Here's how the part is built. I have some questions about the finished solid (model axes, mm). A direction names the side the tool comes from. Give positions to 0.01 mm unless a question says otherwise; leave off trailing zeros. Order: outer loops, then holes, each group sorted by start corner. A loop starts at its lowest first (then second) coordinate and runs counter-clockwise, first axis right, second up. Notation, with made-up numbers: M 67,78.25 L 96,78.25 A17 ccw 96,95.25 Z; hole C -23,-10 d8. An arc over 180 degrees is marked long. One line per item, written item: value. Start each with the question number.
Autodesk Inventor part; units mm, degrees
ref_plane "YZ Plane" through (0, 0, 0) normal (1, 0, 0) x (0, 1, 0)
ref_plane "XZ Plane" through (0, 0, 0) normal (0, 1, 0) x (-1, 0, 0)
ref_plane "XY Plane" through (0, 0, 0) normal (0, 0, 1) x (1, 0, 0)
sketch "Sketch1" plane through (0, 0, 0) normal (0, 1, 0) x (-1, 0, 0)
  circle A0 centre (0, 0) radius 14
  dimension "d0" = 28
extrude "Extrusion1" add sketch "Sketch1" along normal blind 19
sketch "Sketch3" plane through (0, 19, 0) normal (0, 1, 0) x (1, 0, 0)
  circle A0 centre (0, 0) radius 14
  line L0 (3.5, 13.5554) -> (3.5, 17.5)
  arc A1 (3.5, 17.5) -> (-3.5, 17.5) centre (0, 17.5) ccw
  line L1 (-3.5, 17.5) -> (-3.5, 13.5554)
  arc A2 (3.5, 13.5554) -> (-3.5, 13.5554) centre (0, 0) ccw
  circle A3 centre (0, 17.5) radius 2
  line L2 (-3.5, -13.5554) -> (-3.5, -17.5)
  arc A4 (-3.5, -17.5) -> (3.5, -17.5) centre (0, -17.5) ccw
  line L3 (3.5, -17.5) -> (3.5, -13.5554)
  arc A5 (-3.5, -13.5554) -> (3.5, -13.5554) centre (0, 0) ccw
  circle A6 centre (0, -17.5) radius 2
  circle A7 centre (-8, 0) radius 4.5
  dimension "d8" = 9
  dimension "d9" = 8
extrude "Extrusion3" add sketch "Sketch3" along normal blind 1.5 contours A7
sketch "Sketch4" plane through (-8, 20.5, 0) normal (0, 1, 0) x (1, 0, 0)
  circle A0 centre (0, 0) radius 4.5
  circle A1 centre (0, 0) radius 2.5
  point P0 (8, 0)
  dimension "d12" = 5
extrude "Extrusion4" add sketch "Sketch4" along normal blind 8.5 contours A1
sketch "Sketch5" plane through (-8, 29, 0) normal (0, 1, 0) x (1, 0, 0)
  circle A0 centre (0, 0) radius 2.5
  circle A1 centre (0, 0) radius 2.5
  line L0 (-1.5, 2) -> (-1.5, -2)
  line L1 (1.5, -2) -> (1.5, 2)
  point P0 (8, 0)
  point P1 (1.5, 2)
  point P2 (1.5, -2)
  dimension "d15" = 1.5
  dimension "d16" = 3
extrude "Extrusion5" cut sketch "Sketch5" against normal blind 6 contours A0 L1 | L0 A0
sketch "Sketch7" plane through (0, 19, 0) normal (0, 1, 0) x (1, 0, 0)
  circle A0 centre (-8, 0) radius 4.5
  circle A1 centre (0, 0) radius 14
  line L0 (0, -17.5) -> (0, 17.5) construction
  line L1 (3.5, -17.5) -> (3.5, 17.5)
  line L2 (-3.5, 17.5) -> (-3.5, -17.5)
  arc A2 (-3.5, -17.5) -> (3.5, -17.5) centre (0, -17.5) ccw
  arc A3 (3.5, 17.5) -> (-3.5, 17.5) centre (0, 17.5) ccw
  circle A4 centre (0, 17.5) radius 2
  circle A5 centre (0, -17.5) radius 2
  point P0 (3.5, -13.5554)
  point P1 (-3.5, -13.5554)
  point P2 (-3.5, 13.5554)
  point P3 (3.5, 13.5554)
  dimension "d24" = 35
  dimension "d25" = 3.5
  dimension "d26" = 4
extrude "Extrusion7" add sketch "Sketch7" against normal blind 1 contours L2 A3 L1 A1 | A1 L1 A2 L2
sketch "Sketch8" plane through (0, 19, 0) normal (0, 1, 0) x (1, 0, 0)
  arc A0 (3.5, -13.5554) -> (3.5, 13.5554) centre (0, 0) ccw
  line L0 (12.1244, 7) -> (16, 7)
  line L1 (16, 7) -> (16, -7)
  line L2 (16, -7) -> (12.1244, -7)
  circle A1 centre (0, 0) radius 14
  point P0 (14.0622, 7)
  point P1 (16, 0)
  point P2 (14, 0)
  dimension "d29" = 7
  dimension "d30" = 7
  dimension "d31" = 2
extrude "Extrusion8" add sketch "Sketch8" against normal blind 17 contours A0 L0 L1 L2
equation "\"d16\" = 2 * d15"
properties part number "28BYJ-48" material "Aluminum 6061"
Item 1: I want a section at B-B on z = 16.5. Write out the boundary of the cut face in (x, y), plus the area to 3 significant figures.
Item 2: Will these pins go through, and if not, where does the flat tip stop? P1, Ø4.5, axis at x = 14.5, z = 0, coming from the -Y side; P2, Ø6.5, axis at x = 0, z = -17.5, coming from the +Y side; P3, Ø1.5, axis at x = 8, y = 13.5, coming from the +Z side; P4, Ø10, axis at y = 15, z = -16, coming from the -X side.
Item 3: We'd pull the mould along X, two halves only. Please class faces 1 (the face through (-0.26, 18.507, 15.517)), 2 (the face through (3.5, 18.5, -15.5)), 3 (the face through (1, 19, 0)): +X half, -X half, draft (parallel to the pull), parting line (faces both ways), or undercut.
Item 4: I want a section at A-A on x = 0. Write out the boundary of the cut face in (y, z).
Item 5: For faces 4 (the face through (-6, 23, 0)), 5 (the face through (-12.932, 9.367, 5.362)), 6 (the face through (-3.708, 19.74, 1.352)), 7 (the face through (3.5, 18.5, 15.6)), 8 (the face through (-3.5, 18.5, 15.5)), which set-ups out of +Z, -Z, +X, -X, +Y, -Y let a thin tool reach every point of the face, with its end or its side?
Item 6: I want a section at C-C on x = -8. Write out the boundary of the cut face in (y, z), plus the area to 3 significant figures.
Item 7: Please list where these lines run through material, in increasing order: probe 1 along Z at (x, y) = (0, 18.65); probe 2 along X at (y, z) = (18.3, 17.5); probe 3 along Y at (x, z) = (-4.5, -1.5). Write a range as [from, to].
Item 8: I want a section at D-D on z = 0. Write out the boundary of the cut face in (x, y).
Answer below:
1. outline: M -3.5,18 L -1.73,18 L -1.73,19 L -3.5,19 Z; M 1.73,18 L 3.5,18 L 3.5,19 L 1.73,19 Z
1. area: 3.54 mm²
2. P1: stops at y = 0
2. P2: stops at y = 19
2. P3: stops at z = 11.98
2. P4: stops at x = -8.66
3. face 1: undercut
3. face 2: +X half
3. face 3: draft
4. outline: M 0,-14 L 18,-14 L 18,-15.5 L 19,-15.5 L 19,15.5 L 18,15.5 L 18,14 L 0,14 Z; M 18,-21 L 19,-21 L 19,-19.5 L 18,-19.5 Z; M 18,19.5 L 19,19.5 L 19,21 L 18,21 Z
5. face 4: +Z, -Z, +X, +Y
5. face 5: -Y
5. face 6: +Y
5. face 7: +Z, +X, +Y, -Y
5. face 8: +Z, -X, +Y, -Y
6. outline: M 0,-11.49 L 19,-11.49 L 19,-4.5 L 20.5,-4.5 L 20.5,-2.5 L 29,-2.5 L 29,2.5 L 20.5,2.5 L 20.5,4.5 L 19,4.5 L 19,11.49 L 0,11.49 Z
6. area: 493 mm²
7. probe 1: z = [-21, -19.5], [-15.5, 15.5], [19.5, 21]
7. probe 2: x = [-3.5, -2], [2, 3.5]
7. probe 3: y = [0, 20.5]
8. outline: M -14,0 L 14,0 L 14,2 L 16,2 L 16,19 L -3.5,19 L -3.5,20.5 L -5.5,20.5 L -5.5,23 L -6.5,23 L -6.5,29 L -9.5,29 L -9.5,23 L -10.5,23 L -10.5,20.5 L -12.5,20.5 L -12.5,19 L -14,19 Z
